Autodesk Inventor part; units mm, degrees
ref_plane "YZ Plane" through (0, 0, 0) normal (1, 0, 0) x (0, 1, 0)
ref_plane "XZ Plane" through (0, 0, 0) normal (0, 1, 0) x (-1, 0, 0)
ref_plane "XY Plane" through (0, 0, 0) normal (0, 0, 1) x (1, 0, 0)
sketch "Sketch1" plane through (0, 0, 0) normal (0, 0, 1) x (1, 0, 0)
  circle A0 centre (0, 0) radius 4
  dimension "Diameter" = 8
extrude "Extrusion1" add sketch "Sketch1" along normal blind 45
sketch "Sketch2" plane through (0, 0, 45) normal (0, 0, 1) x (1, 0, 0)
  circle A0 centre (0, 0) radius 4
  circle A1 centre (0, 0) radius 6.5
  dimension "Head_Diameter" = 13
extrude "Extrusion2" add sketch "Sketch2" along normal blind 8 contours A0 | A1
sketch "Sketch3" plane through (0, 0, 53) normal (0, 0, 1) x (1, 0, 0)
  circle A0 centre (0, 0) radius 6.5
  circle A1 centre (0, 0) radius 3.4641 construction
  line L0 (0, 3.4641) -> (3, 1.7321)
  line L1 (3, -1.7321) -> (3, 1.7321)
  line L2 (0, 3.4641) -> (-3, 1.7321)
  line L3 (-3, -1.7321) -> (-3, 1.7321)
  line L4 (-3, -1.7321) -> (0, -3.4641)
  line L5 (3, -1.7321) -> (0, -3.4641)
  dimension "Hex_Width" = 6
extrude "Extrusion3" cut sketch "Sketch3" against normal blind 4 contours L0 L1 L5 L4 L3 L2
thread "Thread1"
chamfer "Chamfer1" distance 0.8 angle 45 2 edges at (-6.5, 0, 53) (-4, 0, 0)
equation "\"d12\" = Chamfer"
equation "\"ThreadLength\" = 16"
properties part number "SCREW,SOCKET HD,P,12.9,M8X1.25X45MM"
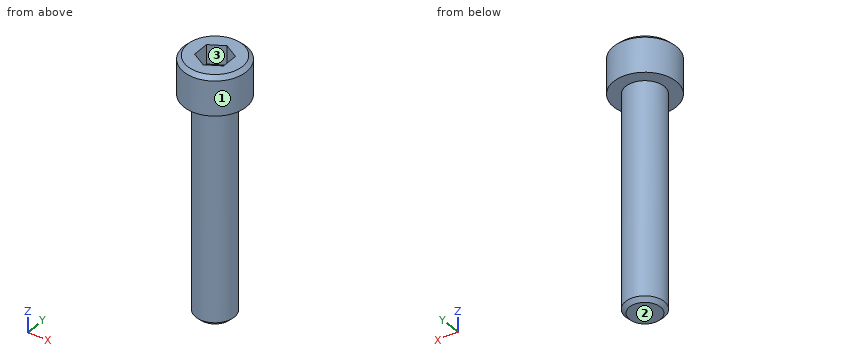
Model file for the job. Use its own axes, mm. Face numbers are marked on the shaded views. Give positions to 0.01 mm unless a question says otherwise; leave off trailing zeros. Loops run counter-clockwise (first coordinate to the right, second up) from the corner with the lowest first, then second, coordinate; pieces in that order, holes last. Notation, with made-up numbers: (66, -18) - (97, -18) arc R28 ccw to (97, 11) - close; hole circle Ø11 at (-8.75, 21). An arc over 180 degrees is marked (long way). One line per item, written item: value. Start each with the question number.
1. Probe L1, parallel to Y at x = 0, z = 3; L2, parallel to Z at x = -1.25, y = -1.5; L3, parallel to Z at x = -1, y = 5. List the from-to ranges inside material, lowest first. Write a range as from..to.
2. Slice it at B-B (z = 33.5). List the corners of the cut face in (x, y).
3. Pin check, flat tips, straight feed: pin 1 (5 mm diameter, centred on y = -5, z = 40, fed in from +X); pin 2 (2 mm diameter, centred on x = 3.5, z = 25.5, fed in from +Y); pin 3 (1.5 mm diameter, centred on x = -4, z = 46.5, fed in from -Y). Stop position of each tip, or through.
4. Pull direction Y, two halves, no side cores. Call the marked faces 1, 2 and 3: pulls with the +Y half, pulls with the -Y half, needs draft (parallel to the pull), parting line crosses it, or undercut.
5. Slice it at A-A (y = 0). List the corners of the cut face in (x, z).
Solution:
1. L1: y = -4..4
1. L2: z = 0..49
1. L3: z = 45..53
2. outline: circle Ø8 at (0, 0)
3. pin 1: stops at x = 3.12
3. pin 2: stops at y = 3.12
3. pin 3: stops at y = -5.63
4. face 1: parting line crosses it
4. face 2: needs draft
4. face 3: undercut
5. outline: (-6.5, 45) - (-4, 45) - (-4, 0.8) - (-3.2, 0) - (3.2, 0) - (4, 0.8) - (4, 45) - (6.5, 45) - (6.5, 52.2) - (5.7, 53) - (3, 53) - (3, 49) - (-3, 49) - (-3, 53) - (-5.7, 53) - (-6.5, 52.2) - close
